The model under review builds one solid part; all positions refer to its coordinate system, in mm. A direction names the side the tool comes from. Round coordinates to 2 decimals unless told otherwise and drop trailing zeros. Order: outer loops, then holes, each group sorted by start corner. A loop starts at its lowest first (then second) coordinate and runs counter-clockwise, first axis right, second up. Notation, with made-up numbers: M 84,31.5 L 140,31.5 A30 cw 140,66.5 Z; hole C 54.25,24.25 d1. An arc over 180 degrees is marked long. Use a Markdown table: item, result. Add a question column.
1. Consider section A-A on x = 55. State the section outline as (y, z) points, then the cut area to 3 significant figures.
2. Insertion check: P1, Ø1.5, axis at x = 49.5, z = 29.5, coming from the +Y side; P2, Ø0.7, axis at x = 59, z = 0.5, coming from the +Y side; P3, Ø16.5, axis at x = 74.5, z = 36, coming from the -Y side. Each pin has a flat end and moves straight along its axis. Give the tip position at first contact, or say it passes through.
3. The part is to be moulded in two halves that separate along X. For faces 4 (the flat face through (65, -43, 57.4)), 5 (the flat face through (0, 1, 9)), 6 (the flat face through (66.896, 6.328, 1.183)), 7 (the flat face through (54.56, 0.58, 1.18)), say which applies: +X half, -X half, draft (parallel to the pull), parting line (faces both ways), or undercut.
4. For faces 1 (the flat face through (63, -45, 30)), 2 (the flat face through (51, 4, 2.4)), 3 (the flat face through (50, -36, 0)), list the 3-axis set-ups (+Z, -Z, +X, -X, +Y, -Y) from which the entire face can be reached by the end or side of a thin tool; tool diameter is ignored.
5. Consider section D-D on y = -35. State the section outline as (x, z) points, then the cut area to 3 significant figures.
6. Consider section C-C on x = 106. State the section outline as (y, z) points.
7. Consider section B-B on y = 13. State the section outline as (x, z) points, then the cut area to 3 significant figures.
8. To check wall thickness, follow probe 1 along Y at (x, z) = (73, 12.5); probe 2 along Z at (x, y) = (14.5, -48.5); probe 3 along X at (y, z) = (25.5, 7.5). State the ranges of each line that lie inside material, in increasing order.
from build123d import *

# Parameters (mm, degrees)
PAD002_DEPTH = 2.4
PAD003_DEPTH = 20
PAD004_DEPTH = 35


with BuildPart() as part:
    # Sketch007 → Pad002 (new body)
    with BuildSketch(Plane.XY):
        Polygon((0, 55), (0, -55), (130, -55), (130, -41), (2, 55), align=None)
        Polygon((14, 31), (14, -29), (94, -29), align=None, mode=Mode.SUBTRACT)
    extrude(amount=PAD002_DEPTH)

    # Sketch008 → Pad003 (join)
    with BuildSketch(Plane.XY.offset(2.4)):
        Polygon((2, 55), (0, 55), (0, -45), (128, -45), (128, -55), (130, -55), (130, -41), (2, -41), align=None)
    extrude(amount=PAD003_DEPTH)

    # Sketch009 → Pad004 (join)
    with BuildSketch(Plane.XY.offset(22.4)):
        Polygon((0, -45), (128, -45), (128, -55), (130, -55), (130, -41), (0, -41), align=None)
    extrude(amount=PAD004_DEPTH)


solid = part.part
Answer block:
| question | item | result |
|---|---|---|
| 1 | outline | M -55,0 L -29,0 L -29,2.4 L -41,2.4 L -41,57.4 L -45,57.4 L -45,2.4 L -55,2.4 Z; M 0.25,0 L 15.25,0 L 15.25,2.4 L 0.25,2.4 Z |
| 1 | area | 318 mm^2 |
| 2 | P1 | y = -41 |
| 2 | P2 | y = 12.51 |
| 2 | P3 | y = -45 |
| 3 | face 4 | draft |
| 3 | face 5 | -X half |
| 3 | face 6 | +X half |
| 3 | face 7 | undercut |
| 4 | face 1 | +Z, -X, -Y |
| 4 | face 2 | +Z, +X, +Y |
| 4 | face 3 | -Z, +X, -X, +Y, -Y |
| 5 | outline | M 0,0 L 122,0 L 122,2.4 L 2,2.4 L 2,22.4 L 0,22.4 Z |
| 5 | area | 333 mm^2 |
| 6 | outline | M -55,0 L -23,0 L -23,2.4 L -41,2.4 L -41,57.4 L -45,57.4 L -45,2.4 L -55,2.4 Z |
| 7 | outline | M 0,0 L 14,0 L 14,2.4 L 2,2.4 L 2,22.4 L 0,22.4 Z; M 38,0 L 58,0 L 58,2.4 L 38,2.4 Z |
| 7 | area | 122 mm^2 |
| 8 | probe 1 | -45 to -41 |
| 8 | probe 2 | 0 to 2.4 |
| 8 | probe 3 | 0 to 2 |
